from build123d import *

# Parameters (mm, degrees)
CYLINDER021_R     = 3.5
CYLINDER021_DEPTH = 6
CYLINDER017_R     = 6
CYLINDER017_DEPTH = 4
CYLINDER015_R     = 9
CYLINDER015_DEPTH = 12
FILLET012_R       = 2


with BuildPart() as knob_cut003:
    # Cylinder021 → Cylinder021 (new body)
    with BuildSketch(Plane.XY.offset(10)):
        Circle(CYLINDER021_R)
    extrude(amount=CYLINDER021_DEPTH)


with BuildPart() as knob_cut001:
    # Cylinder017 → Cylinder017 (new body)
    with BuildSketch(Plane.XY.offset(6)):
        Circle(CYLINDER017_R)
    extrude(amount=CYLINDER017_DEPTH)


with BuildPart() as knob003:
    # Cylinder015 → Cylinder015 (new body)
    with BuildSketch(Plane.XY.offset(6)):
        Circle(CYLINDER015_R)
    extrude(amount=CYLINDER015_DEPTH)

    # Cut020: cut KNOB_cut001
    add(knob_cut001.part, mode=Mode.SUBTRACT)

    # Cut021: cut KNOB_cut003
    add(knob_cut003.part, mode=Mode.SUBTRACT)

    # Fillet012
    fillet012_edges = [knob003.edges().sort_by_distance(p)[0] for p in [
        (-9, 0, 18),
    ]]
    fillet(fillet012_edges, radius=FILLET012_R)


solid = knob003.part
Model file for the job. Use its own axes, mm. A direction names the side the tool comes from. Round coordinates to 2 decimals unless told otherwise and drop trailing zeros. Order: outer loops, then holes, each group sorted by start corner. A loop starts at its lowest first (then second) coordinate and runs counter-clockwise, first axis right, second up.
(1) Pin check, flat tips, straight feed: pin 1 (3.5 mm diameter, centred on x = -1.5, y = 1.5, fed in from -Z); pin 2 (1 mm diameter, centred on y = -1.5, z = 15.5, fed in from -X); pin 3 (1 mm diameter, centred on x = -7, y = -5, fed in from +Z). Stop position of each tip, or through.
(2) 3-axis set-ups, long thin cutter, end or side, ignore diameter. For faces 1 (the face through (3, -3, 10)), 2 (the face through (0, 0, 18)): which of +Z, -Z, +X, -X, +Y, -Y reach the whole face in a straight line?
(3) Band-saw the part on D-D (z = 16.5). List the corners of the cut face in (x, y), then the cut area to 3 significant figures.
(4) Band-saw the part on C-C (z = 15.25). List the corners of the cut face in (x, y), then the cut area to 3 significant figures.
(5) Drill centre lines: line 1 (Y direction, x = 0, z = 14.1); line 2 (Y direction, x = 0, z = 7.4); line 3 (Z direction, x = -3.75, y = 0.75). Where is each one in solid material? Low to high.
(6) Pull direction X, two halves, no side cores. Call faces 3 (the face through (0, 0, 16)), 4 (the face through (2, -6, 6)), 5 (the face through (-1.172, 8.923, 10.93)): released by +X, released by -X, zero draft, split by the parting line, or undercut.
(7) Band-saw the part on A-A (x = 0). List the corners of the cut face in (y, z), then the cut area to 3 significant figures.
Verdict:
1. pin 1: stops at z = 10
1. pin 2: stops at x = -8.94
1. pin 3: stops at z = 17.67
2. face 1: -Z
2. face 2: +Z, +X, -X, +Y, -Y
3. outline: circle Ø17.87 at (0, 0)
3. area: 251 mm2
4. outline: circle Ø18 at (0, 0); hole circle Ø7 at (0, 0)
4. area: 216 mm2
5. line 1: y = -9 to -3.5, 3.5 to 9
5. line 2: y = -9 to -6, 6 to 9
5. line 3: z = 10 to 18
6. face 3: undercut
6. face 4: zero draft
6. face 5: split by the parting line
7. outline: (-9, 6) - (-6, 6) - (-6, 10) - (-3.5, 10) - (-3.5, 16) - (3.5, 16) - (3.5, 10) - (6, 10) - (6, 6) - (9, 6) - (9, 16) arc R2 ccw to (7, 18) - (-7, 18) arc R2 ccw to (-9, 16) - close
7. area: 124 mm2
